Check sheet for the modelled part. Datum: model origin and axes. Units: mm. Give positions to 0.01 mm unless a question says otherwise; leave off trailing zeros. Order: outer loops, then holes, each group sorted by start corner. A loop starts at its lowest first (then second) coordinate and runs counter-clockwise, first axis right, second up. Notation, with made-up numbers: M 82.5,49.5 L 91.5,49.5 A16 cw 91.5,60.5 Z; hole C 28.5,1.5 d7. An arc over 180 degrees is marked long. Answer in a Markdown table with one row per item. Add a question column.
from build123d import *

# Parameters (mm, degrees)
F0_R     = 1.5
F0_W     = 27
F0_H     = 5
F2_DEPTH = 3.5


with BuildPart() as f2:
    # F0 (on Top) → F2 (new body)
    with BuildSketch(Plane.XY):
        Polygon((-160, 103.5), (-180, 103.5), (-180, -103.5), (-141, -103.5), (-141, -114.5), (-72, -114.5), (-45, -114.5), (144, -114.5), (144, -103.5), (147, -103.5), (147, -109.5), (160, -109.5), (160, -103.5), (180, -103.5), (180, 103.5), (160, 103.5), (160, 109.5), (147, 109.5), (147, 103.5), (-147, 103.5), (-147, 109.5), (-160, 109.5), align=None)
        with Locations((150.5, -106.5)):
            Circle(F0_R, mode=Mode.SUBTRACT)
        with Locations((156.5, -106.5)):
            Circle(F0_R, mode=Mode.SUBTRACT)
        with Locations((-156.5, 106.5)):
            Circle(F0_R, mode=Mode.SUBTRACT)
        with Locations((-150.5, 106.5)):
            Circle(F0_R, mode=Mode.SUBTRACT)
        with Locations((150.5, 106.5)):
            Circle(F0_R, mode=Mode.SUBTRACT)
        with Locations((156.5, 106.5)):
            Circle(F0_R, mode=Mode.SUBTRACT)
        with Locations((-58.5, -117)):
            Rectangle(F0_W, F0_H)
    extrude(amount=F2_DEPTH)


solid = f2.part
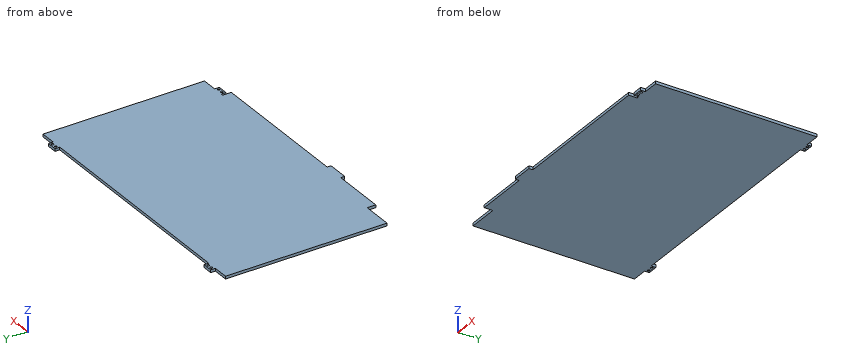
Q1. Go/stop test with flat-tipped pins: pin 1 (2.5 mm diameter, centred on x = 150.5, y = 106.5, fed in from +Z); pin 2 (1.8 mm diameter, centred on y = -106, z = 1.5, fed in from +X); pin 3 (1 mm diameter, centred on x = 152, z = 2.5, fed in from -Y); pin 4 (4 mm diameter, centred on x = -29, y = 32, fed in from -Z). Record where each tip stops, or that it passes through.
Q2. Cross-section at C-C (x = -125). Record the boundary of the cut face in (y, z).
Q3. Thickness scan on probe 1 along Y at (x, z) = (150.5, 1.7); probe 2 along X at (y, z) = (106.5, 2.25); probe 3 along Y at (x, z) = (-150.5, 1). Record the ranges inside material, lowest first.
Q4. Cross-section at A-A (z = 1.85). State how many separate pieces and enclosed holes the cut face has, and give its area (3 significant figures).
Q5. Cross-section at B-B (x = -64). Record the boundary of the cut face in (y, z).
Values follow:
| question | item | result |
|---|---|---|
| 1 | pin 1 | through |
| 1 | pin 2 | x = 160 |
| 1 | pin 3 | y = -109.5 |
| 1 | pin 4 | z = 0 |
| 2 | outline | M -114.5,0 L 103.5,0 L 103.5,3.5 L -114.5,3.5 Z |
| 3 | probe 1 | -109.5 to -108, -105 to 105, 108 to 109.5 |
| 3 | probe 2 | -160 to -158, -155 to -152, -149 to -147, 147 to 149, 152 to 155, 158 to 160 |
| 3 | probe 3 | -103.5 to 105, 108 to 109.5 |
| 4 | separate pieces | 1 |
| 4 | enclosed holes | 6 |
| 4 | area | 78,000 mm² |
| 5 | outline | M -119.5,0 L 103.5,0 L 103.5,3.5 L -119.5,3.5 Z |
